Here's how the part is built. I have some questions about the finished solid (model axes, mm). A direction names the side the tool comes from. Coordinates: 2 decimals unless noted, no trailing zeros. Loops run counter-clockwise (first coordinate to the right, second up) from the corner with the lowest first, then second, coordinate; pieces in that order, holes last. Notation, with made-up numbers: (8, 18.5) -> (45, 18.5) arc R26 ccw to (45, 34.5) -> close; hole circle Ø8 at (-25, 67). An arc over 180 degrees is marked (long way). Answer as a JSON object with one key per item and string values. Group by question number.
1) I want a section at C-C (y = 24). Write out the boundary of the cut face in (x, z).
2) I want a section at D-D (y = 78). Write out the boundary of the cut face in (x, z), then the cut area to 3 significant figures.
3) Which directions (+Z, -Z, +X, -X, +Y, -Y) give clear straight access to the entire face, cutting with the end or side of a thin tool? Please do faces 4 (the flat face through (-21, 0, -7)), 5 (the flat face through (4, 76.2, 0)).
4) I need wall thicknesses on probe 1 along X at (y, z) = (45.5, 0); probe 2 along X at (y, z) = (90.75, 0); probe 3 along Z at (x, y) = (0.5, 11.5). Which ranges of each line are inside material? Lowest first, please. Write a range as [from, to].
5) I want a section at B-B (x = 0). Write out the boundary of the cut face in (y, z).
6) I want a section at A-A (z = 0). Write out the boundary of the cut face in (x, y).
7) If we mould it in two halves opening along Z, with no side actions, what happens to faces 1 (the cylindrical face through (0.767, 85.592, -2.435)), 2 (the cylindrical face through (9.78, 46.96, -23.58)), 3 (the flat face through (0, 95.25, -5))? For each: +Z half, -Z half, draft (parallel to the pull), parting line (faces both ways), or undercut.
8) I'm going to push flat-ended pins straight in: pin 1 (2 mm diameter, centred on x = 19, z = 4, fed in from -Y); pin 2 (8 mm diameter, centred on x = -2, y = 52.5, fed in from -Z); pin 3 (10 mm diameter, centred on y = 11, z = 15.5, fed in from +X); pin 4 (5 mm diameter, centred on x = -8, z = -1.5, fed in from -Y). Where does each tip first touch, or does it pass through?
```python
from build123d import *

# Parameters (mm, degrees)
SKETCH1_R                   = 25.527
SKETCH1_R_2                 = 19.177
BOSS_EXTRUDE1_DEPTH         = 76.2
SKETCH2_R                   = 25.527
BOSS_EXTRUDE2_DEPTH         = 19.05
TAP_DRILL_FOR_1_4_20_TAP1_D = 5.1054
FILLET1_R                   = 2.54


with BuildPart() as part:
    # Sketch1 → Boss-Extrude1 (new body)
    with BuildSketch(Plane(origin=(0, 0, 0), x_dir=(1, 0, 0), z_dir=(0, 1, 0))):
        with Locations(Location((0, 0, 0), (0, 0, 90))):
            Circle(SKETCH1_R)
        with Locations(Location((0, 0, 0), (0, 0, 90))):
            Circle(SKETCH1_R_2, mode=Mode.SUBTRACT)
    extrude(amount=BOSS_EXTRUDE1_DEPTH)

    # Sketch2 → Boss-Extrude2 (add)
    with BuildSketch(Plane(origin=(0, 76.2, 0), x_dir=(1, 0, 0), z_dir=(0, 1, 0))):
        with Locations(Location((0, 0, 0), (0, 0, 90))):
            Circle(SKETCH2_R)
    extrude(amount=BOSS_EXTRUDE2_DEPTH)

    # Tap Drill for 1/4-20 Tap1 (through all)
    with Locations(Plane.ZX.offset(95.25)):
        with Locations((0, 0)):
            Hole(TAP_DRILL_FOR_1_4_20_TAP1_D / 2)

    # Fillet1
    fillet1_edges = [part.edges().sort_by_distance(p)[0] for p in [
        (0, 0, 19.177),
    ]]
    fillet(fillet1_edges, radius=FILLET1_R)


solid = part.part
```
Determined:
{
 "1": {"outline": "circle Ø51.05 at (0, 0); hole circle Ø38.35 at (0, 0)"},
 "2": {"outline": "circle Ø51.05 at (0, 0); hole circle Ø5.11 at (0, 0)", "area": "2,030 mm^2"},
 "3": {"face 4": "+Z, -Z, +X, -X, -Y", "face 5": "-Y"},
 "4": {"probe 1": "[-25.53, -19.18], [19.18, 25.53]", "probe 2": "[-25.53, -2.55], [2.55, 25.53]", "probe 3": "[-25.52, -19.17], [19.17, 25.52]"},
 "5": {"outline": "(0, -25.53) -> (95.25, -25.53) -> (95.25, -2.55) -> (76.2, -2.55) -> (76.2, -19.18) -> (2.54, -19.18) arc R2.54 ccw to (0, -21.72) -> close; (0, 21.72) arc R2.54 ccw to (2.54, 19.18) -> (76.2, 19.18) -> (76.2, 2.55) -> (95.25, 2.55) -> (95.25, 25.53) -> (0, 25.53) -> close"},
 "6": {"outline": "(-25.53, 0) -> (-21.72, 0) arc R2.54 ccw to (-19.18, 2.54) -> (-19.18, 76.2) -> (-2.55, 76.2) -> (-2.55, 95.25) -> (-25.53, 95.25) -> close; (2.55, 76.2) -> (19.18, 76.2) -> (19.18, 2.54) arc R2.54 ccw to (21.72, 0) -> (25.53, 0) -> (25.53, 95.25) -> (2.55, 95.25) -> close"},
 "7": {"face 1": "undercut", "face 2": "parting line", "face 3": "draft"},
 "8": {"pin 1": "y = 0.36", "pin 2": "z = -25.53", "pin 3": "x = 23.27", "pin 4": "y = 76.2"}
}
